```python
from build123d import *

# Parameters (mm, degrees)
SKETCH1_R           = 1.6
SKETCH1_W           = 30.70266837
SKETCH1_H           = 18.457088441
SKETCH1_W_2         = 23.2
SKETCH1_H_2         = 12.2
BOSS_EXTRUDE5_DEPTH = 6.5


with BuildPart() as part:
    # Sketch1 → Boss-Extrude5 (new body)
    # profile 1 of 2: a face of its own
    with BuildSketch(Plane(origin=(0, 0, 0), x_dir=(1, 0, 0), z_dir=(0, 1, 0))):
        Polygon((23.208363186, 35.61697891), (23.208363186, 32.900104101), (31.932950893, 32.900104101), (31.932950893, 35.61697891), (36.695280427, 35.61697891), (36.695280427, 30.61697891), (18.217441835, 30.61697891), (18.217441835, 35.61697891), align=None)
        with Locations(Location((20.712902511, 33.11697891, 0), (0, 0, 90))):
            Circle(SKETCH1_R, mode=Mode.SUBTRACT)
        with Locations(Location((34.31411566, 33.11697891, 0), (0, 0, 90))):
            Circle(SKETCH1_R, mode=Mode.SUBTRACT)
    # profile 2 of 2: a face of its own
    with BuildSketch(Plane(origin=(0, 0, 0), x_dir=(1, 0, 0), z_dir=(0, 1, 0))):
        with Locations((27.63237184, 21.38843469)):
            Rectangle(SKETCH1_W, SKETCH1_H)
        with Locations((27.508406256, 21.602944359)):
            Rectangle(SKETCH1_W_2, SKETCH1_H_2, mode=Mode.SUBTRACT)
    extrude(amount=BOSS_EXTRUDE5_DEPTH)


solid = part.part
```
Here's how the part is built. I have some questions about the finished solid (model axes, mm). A direction names the side the tool comes from. Round coordinates to 2 decimals unless told otherwise and drop trailing zeros. Loops run counter-clockwise (first coordinate to the right, second up) from the corner with the lowest first, then second, coordinate; pieces in that order, holes last. Notation, with made-up numbers: (42.25, 46.25) -> (54.25, 46.25) arc R14 ccw to (54.25, 50.25) -> close; hole circle Ø5 at (27, 4). An arc over 180 degrees is marked (long way). Answer as CSV lines item,"result".
1. If I drill on L1, parallel to Z at x = 31.5, y = 3.5; L2, parallel to X at y = 5.75, z = -23; L3, parallel to X at y = 1.5, z = -33.25, over which ranges is the centre line in solid material (lowest first)?
Final values:
L1,"z = -32.9 to -27.7, -15.5 to -12.16"
L2,"x = 12.28 to 15.91, 39.11 to 42.98"
L3,"x = 18.22 to 19.12, 22.31 to 23.21, 31.93 to 32.72, 35.91 to 36.7"
2. If we section it at A-A on x = 38.5: Please give me the cut outline in (y, z).
Final values:
outline,"(0, -30.62) -> (6.5, -30.62) -> (6.5, -27.7) -> (0, -27.7) -> close; (0, -15.5) -> (6.5, -15.5) -> (6.5, -12.16) -> (0, -12.16) -> close"
3. If we section it at C-C on z = -34: Please give me the cut outline in (x, y).
Final values:
outline,"(18.22, 0) -> (19.38, 0) -> (19.38, 6.5) -> (18.22, 6.5) -> close; (22.05, 0) -> (23.21, 0) -> (23.21, 6.5) -> (22.05, 6.5) -> close; (31.93, 0) -> (32.98, 0) -> (32.98, 6.5) -> (31.93, 6.5) -> close; (35.65, 0) -> (36.7, 0) -> (36.7, 6.5) -> (35.65, 6.5) -> close"
4. Which directions (+Z, -Z, +X, -X, +Y, -Y) give clear straight access to the entire face, cutting with the end or side of a thin tool? Please do faces 1 (the face through (39.108, 3, -22)), 2 (the face through (36.695, 3, -33)), 3 (the face through (31.933, 3, -34)).
Final values:
face 1,"+Y, -Y"
face 2,"-Z, +X, +Y, -Y"
face 3,"-Z, +Y, -Y"
5. Thinking about a two-plate mould opening in X: for faces 4 (the face through (34, 3, -35.617)), 5 (the face through (27, 3, -27.703)), 6 (the face through (20.232, 3.204, -34.643)), 7 (the face through (18.217, 3, -33)), which applies, released by +X, released by -X, zero draft, split by the parting line, or undercut?
Final values:
face 4,"zero draft"
face 5,"undercut"
face 6,"undercut"
face 7,"released by -X"
6. For pin 1 (2 mm diameter, centred on x = 29.5, y = 3.5, fed in from -Z); pin 2 (3 mm diameter, centred on x = 14, y = 3.5, fed in from -Z); pin 3 (3 mm diameter, centred on y = 1.5, z = -33.5, fed in from -X), each with a flat end and sliding along its axis, tell me the tip position at first contact or that it passes through.
Final values:
pin 1,"stops at z = -32.9"
pin 2,"stops at z = -30.62"
pin 3,"stops at x = 18.22"
7. If we section it at D-D on y = 4.5: Please give me the cut outline in (x, z).
Final values:
outline,"(12.28, -30.62) -> (18.22, -30.62) -> (18.22, -35.62) -> (23.21, -35.62) -> (23.21, -32.9) -> (31.93, -32.9) -> (31.93, -35.62) -> (36.7, -35.62) -> (36.7, -30.62) -> (42.98, -30.62) -> (42.98, -12.16) -> (12.28, -12.16) -> close; hole (15.91, -27.7) -> (39.11, -27.7) -> (39.11, -15.5) -> (15.91, -15.5) -> close; hole circle Ø3.2 at (20.71, -33.12); hole circle Ø3.2 at (34.31, -33.12)"
8. If we section it at B-B on z = -23.25: Please give me the cut outline in (x, y), plus the area to 3 significant figures.
Final values:
outline,"(12.28, 0) -> (15.91, 0) -> (15.91, 6.5) -> (12.28, 6.5) -> close; (39.11, 0) -> (42.98, 0) -> (42.98, 6.5) -> (39.11, 6.5) -> close"
area,"48.8 mm^2"
